The figure shows three views and two pictorial views of one solid part (mm, origin at its lowest corner). Answer the questions. A direction names the side the tool comes from. Give positions to 0.01 mm unless a question says otherwise; leave off trailing zeros. Write each loop counter-clockwise with the first axis right and the second up, starting at its lowest first coordinate (ties: lowest second). Pieces come first, ordered by that corner, then holes. Notation, with made-up numbers: (47.25, -30) -> (91.25, -30) arc R31 cw to (91.25, 3) -> close; hole circle Ø3 at (84, 10.25). An arc over 180 degrees is marked (long way). Write item = value, one per line. Start each with the question number.
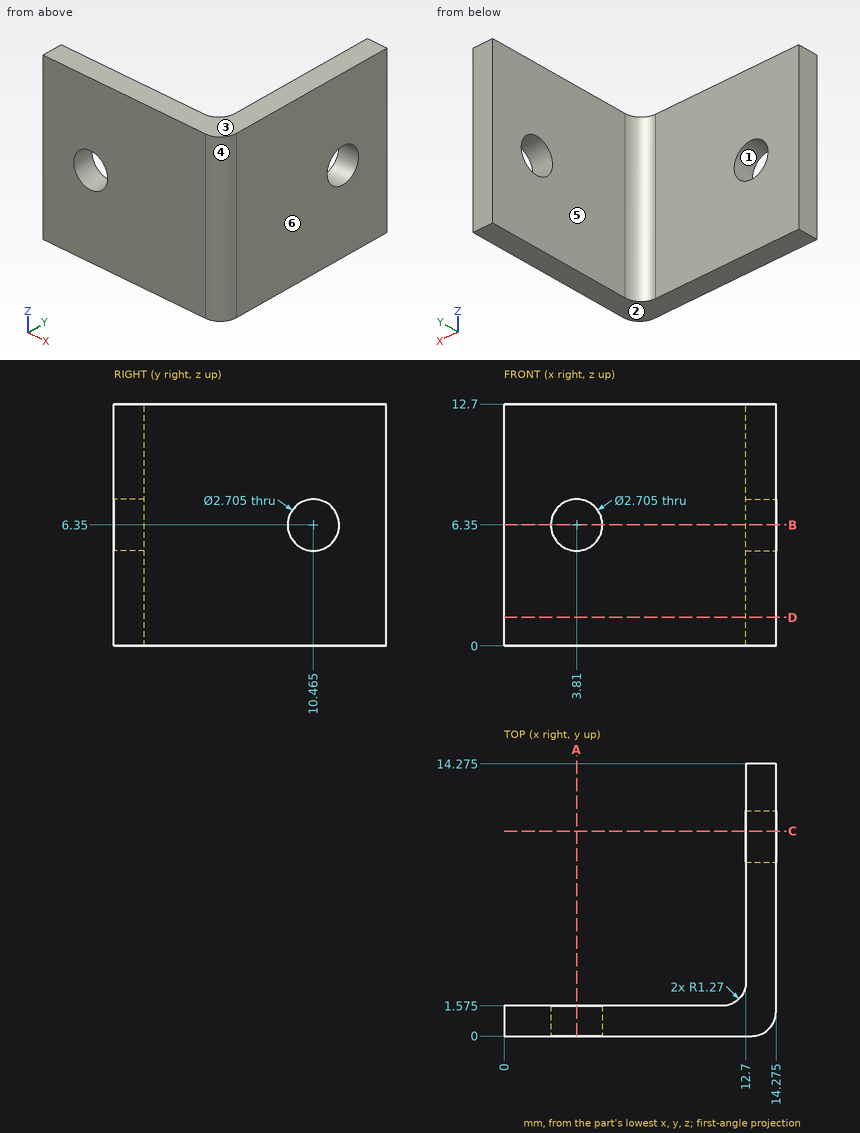
(1) Each of these flat-tipped pins is pushed along its axis until it touches: pin 1 (5.5 mm diameter, centred on x = 8.5, z = 9, fed in from +Y) (3 decimals); pin 2 (3.5 mm diameter, centred on y = 6.5, z = 5, fed in from -X). Where does it stop, or does it pass through?
(2) A cutting plane is placed at B-B, the plane z = 6.35. Write down the section's boundary in (x, y) (1 decimal).
(3) For the marked faces 5 and 6, determine the directions among +Z, -Z, +X, -X, +Y, -Y from which every point of the face is accessible in a straight line to the end or side of a thin tool.
(4) A cutting plane is placed at C-C, the plane y = 10.75. Write down the section's boundary in (x, z) (1 decimal), then the cut area to 3 significant figures.
(5) A cutting plane is placed at A-A, the plane x = 3.81. Write down the section's boundary in (y, z) (1 decimal).
(6) A cutting plane is placed at D-D, the plane z = 1.5. Write down the section's boundary in (x, y) (1 decimal), then the cut area to 3 significant figures.
(7) Find the intervals of material crossed by line 1 along X through (y, z) = (8.75, 2) (1 decimal); line 2 along Y through (x, z) = (7, 1.5) (1 decimal); line 3 along X through (y, z) = (1.5, 7.5) (1 decimal), in increasing order.
(8) Determine the mould class of the marked faces 1, 2, 3 and 4 for opening direction Z: pulls with the +Z half, pulls with the -Z half, needs draft (parallel to the pull), parting line crosses it, or undercut.
Results list:
q1.pin_1 = 1.575
q1.pin_2 = 12.7
q2.outline = (0, 0) -> (2.5, 0) -> (2.5, 1.6) -> (0, 1.6) -> close; (5.2, 0) -> (13, 0) arc R1.3 ccw to (14.3, 1.3) -> (14.3, 9.1) -> (12.7, 9.1) -> (12.7, 2.8) arc R1.3 cw to (11.4, 1.6) -> (5.2, 1.6) -> close; (12.7, 11.8) -> (14.3, 11.8) -> (14.3, 14.3) -> (12.7, 14.3) -> close
q3.face_5 = +Z, -Z, -X, +Y
q3.face_6 = +Z, -Z, +X, +Y, -Y
q4.outline = (12.7, 0) -> (14.3, 0) -> (14.3, 5) -> (12.7, 5) -> close; (12.7, 7.7) -> (14.3, 7.7) -> (14.3, 12.7) -> (12.7, 12.7) -> close
q4.area = 15.8 mm²
q5.outline = (0, 0) -> (1.6, 0) -> (1.6, 5) -> (0, 5) -> close; (0, 7.7) -> (1.6, 7.7) -> (1.6, 12.7) -> (0, 12.7) -> close
q6.outline = (0, 0) -> (13, 0) arc R1.3 ccw to (14.3, 1.3) -> (14.3, 14.3) -> (12.7, 14.3) -> (12.7, 2.8) arc R1.3 cw to (11.4, 1.6) -> (0, 1.6) -> close
q6.area = 42.5 mm²
q7.line_1 = 12.7 to 14.3
q7.line_2 = 0 to 1.6
q7.line_3 = 0 to 3.1, 4.5 to 14.3
q8.face_1 = undercut
q8.face_2 = pulls with the -Z half
q8.face_3 = pulls with the +Z half
q8.face_4 = needs draft
